Verification items for the finished model (mm, model axes). Face numbers are marked on the shaded views. A direction names the side the tool comes from. Coordinates: 2 decimals unless noted, no trailing zeros. Write each loop counter-clockwise with the first axis right and the second up, starting at its lowest first coordinate (ties: lowest second). Pieces come first, ordered by that corner, then holes. Notation, with made-up numbers: (61.5, 7) -> (105.5, 7) arc R20 ccw to (105.5, 13) -> close; hole circle Ø6 at (80, 49). An arc over 180 degrees is marked (long way). Use a Markdown table: item, result. Add a question column.
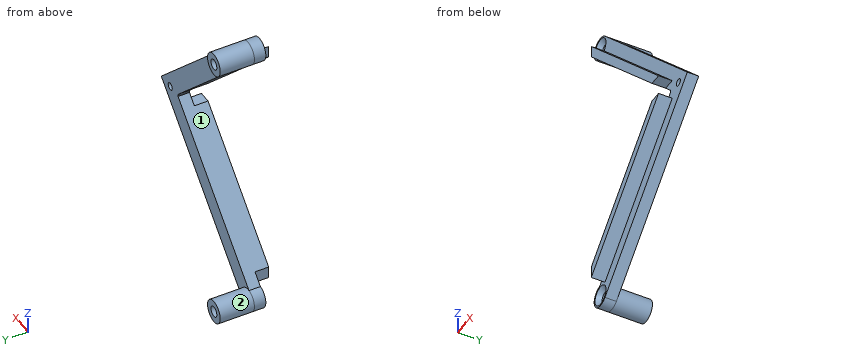
Autodesk Inventor part; units mm, degrees
ref_plane "Work Plane1" through (0, -3.81, 0) normal (0, 1, 0) x (1, 0, 0)
ref_plane "YZ Plane" through (0, 0, 0) normal (1, 0, 0) x (0, 1, 0)
ref_plane "XZ Plane" through (0, 0, 0) normal (0, 1, 0) x (-1, 0, 0)
sketch "Sketch1" plane through (0, 0, 0) normal (0, 1, 0) x (-1, 0, 0)
  line L0 (-41.3092, 0) -> (0, 41.3092)
  circle A0 centre (-36.8191, 0) radius 1.016
  arc A1 (-32.8821, 0) -> (-34.0352, 2.7839) centre (-36.8191, 0) ccw
  line L1 (0, 41.3092) -> (2.2451, 39.0641)
  arc A2 (0, 36.8191) -> (0, 41.3092) centre (2.2451, 39.0641) ccw
  circle A3 centre (2.2451, 39.0641) radius 1.4732
  line L2 (0, 36.8191) -> (-34.0352, 2.7839)
  line L3 (0, 0) -> (-14.0183, 0)
  line L4 (-41.3092, 0) -> (0, -41.3092)
  circle A4 centre (-36.8191, 0) radius 1.016
  arc A5 (-34.0352, -2.7839) -> (-32.8821, 0) centre (-36.8191, 0) ccw
  line L5 (0, -41.3092) -> (2.2451, -39.0641)
  arc A6 (0, -41.3092) -> (0, -36.8191) centre (2.2451, -39.0641) ccw
  circle A7 centre (2.2451, -39.0641) radius 1.4732
  line L6 (0, -36.8191) -> (-34.0352, -2.7839)
  dimension "d0" = 3.175
  dimension "d1" = 58.42
  dimension "d2" = 45
  dimension "d3" = 2.9464
  dimension "d4" = 3.175
  dimension "d5" = 3.937
  dimension "d6" = 2.032
  dimension "d7" = 45
extrude "Extrusion1" add sketch "Sketch1" along normal blind 3.175
sketch "Sketch2" plane through (0, 3.175, 0) normal (0, 1, 0) x (1, 0, 0)
  circle A0 centre (-2.2451, -39.0641) radius 1.4732
  circle A1 centre (-2.2451, -39.0641) radius 3.175
  circle A2 centre (-2.2451, 39.0641) radius 1.4732
  circle A3 centre (-2.2451, 39.0641) radius 3.175
  point P0 (0, 0)
  dimension "d10" = 6.35
  dimension "d11" = 6.35
extrude "Extrusion2" add sketch "Sketch2" along normal blind 9.525
chamfer "Chamfer1" distance 1.27 angle 45 2 edges at (-0.7719, 0, 39.0641) (-0.7719, 0, -39.0641)
sketch "Sketch3" plane through (0, 3.175, 0) normal (0, 1, 0) x (1, 0, 0)
  arc A0 (0, -36.8191) -> (0, -41.3092) centre (-2.2451, -39.0641) ccw
  line L0 (34.0352, -2.7839) -> (0, -36.8191)
  arc A1 (34.0352, 2.7839) -> (34.0352, -2.7839) centre (36.8191, 0) ccw
  line L1 (0, 36.8191) -> (34.0352, 2.7839)
  arc A2 (0, 41.3092) -> (0, 36.8191) centre (-2.2451, 39.0641) ccw
  line L2 (-2.6941, -35.921) -> (32.896, -0.331)
  arc A3 (34.0352, 2.7839) -> (34.0352, -2.7839) centre (36.8191, 0) ccw
  line L3 (32.896, 0.331) -> (-2.6941, 35.921)
  point P0 (0, 0)
  dimension "d17" = 2.54
  dimension "d18" = 2.54
ref_plane "Work Plane1" through (0, -3.81, 0) normal (0, 1, 0) x (1, 0, 0)
extrude "Extrusion3" add sketch "Sketch3" against normal up to surface (3.175 mm away)
sketch "Sketch4" plane through (0, 0, 0) normal (0, -1, 0) x (1, 0, 0)
  line L0 (0, -36.8191) -> (34.0352, -2.7839)
  line L1 (0, 36.8191) -> (34.0352, 2.7839)
  line L2 (-2.6941, -35.921) -> (32.896, -0.331)
  line L3 (-1.6524, -34.8793) -> (32.0954, -1.1315)
  line L4 (32.0954, -1.1315) -> (33.7478, -2.7839)
  line L5 (33.7478, -2.7839) -> (0, -36.5317)
  line L6 (0, -36.5317) -> (-1.6524, -34.8793)
  line L7 (0, 0) -> (11.5163, 0)
  line L8 (-1.6524, 34.8793) -> (32.0954, 1.1315)
  line L9 (32.0954, 1.1315) -> (33.7478, 2.7839)
  line L10 (33.7478, 2.7839) -> (0, 36.5317)
  line L11 (0, 36.5317) -> (-1.6524, 34.8793)
  dimension "d22" = 0.2032
  dimension "d23" = 0.2032
  dimension "d24" = 0.2032
extrude "Extrusion4" add sketch "Sketch4" along normal up to surface (3.81 mm away)
chamfer "Chamfer2" distance 2.3368 angle 45 4 edges at (-1.6524, -1.905, -34.8793) (-1.6524, -1.905, 34.8793) (32.0954, -1.905, 1.1315) (32.0954, -1.905, -1.1315)
properties part number "WIDE SCREEN HOLDER 2SCREEN"
1) Cross-section at B-B on y = 9. Record the boundary of the cut face in (x, z) (3 decimals), then the cut area to 3 significant figures.
2) Thickness scan on L1, parallel to Z at x = -2.5, y = 2.75; L2, parallel to Z at x = 12, y = 1.5; L3, parallel to Z at x = 4.5, y = 2.5. Record the ranges inside material, lowest first.
3) Cross-section at A-A on x = 6. Record the boundary of the cut face in (y, z) (3 decimals).
4) Gauge pin test, flat ends, axial feed: pin 1 (1 mm diameter, centred on x = 1, y = -1.5, fed in from +Z); pin 2 (2.5 mm diameter, centred on x = 36.82, z = 0, fed in from +Y) (3 decimals); pin 3 (1 mm diameter, centred on y = -1.5, z = 34.5, fed in from -X); pin 4 (2.5 mm diameter, centred on x = -2.25, z = 39.06, fed in from -Y). Record the tip position at first contact, or that the pin passes through.
5) Cross-section at C-C on z = 15. Record the boundary of the cut face in (x, y) (3 decimals).
6) Set-up check for the marked faces 1 and 2: record each of +Z, -Z, +X, -X, +Y, -Y from which the full face is reachable in a straight line by a thin tool's end or side.
Returned:
| question | item | result |
|---|---|---|
| 1 | outline | circle Ø6.35 at (-2.245, -39.064); circle Ø6.35 at (-2.245, 39.064); hole circle Ø2.946 at (-2.245, -39.064); hole circle Ø2.946 at (-2.245, 39.064) |
| 1 | area | 49.7 mm² |
| 2 | L1 | z = -42.23 to -40.52, -37.61 to -35.73, 35.73 to 37.61, 40.52 to 42.23 |
| 2 | L2 | z = -29.31 to -21.23, 21.23 to 29.31 |
| 2 | L3 | z = -36.81 to -28.73, 28.73 to 36.81 |
| 3 | outline | (-3.81, -30.532) -> (0, -30.532) -> (0, -35.309) -> (3.175, -35.309) -> (3.175, -27.227) -> (-3.81, -27.227) -> close; (-3.81, 27.227) -> (3.175, 27.227) -> (3.175, 35.309) -> (0, 35.309) -> (0, 30.532) -> (-3.81, 30.532) -> close |
| 4 | pin 1 | stops at z = 36.03 |
| 4 | pin 2 | stops at y = 3.175 |
| 4 | pin 3 | stops at x = 0 |
| 4 | pin 4 | passes through |
| 5 | outline | (18.227, -3.81) -> (21.532, -3.81) -> (21.532, 0) -> (26.309, 0) -> (26.309, 3.175) -> (18.227, 3.175) -> close |
| 6 | face 1 | -X, +Y, -Y |
| 6 | face 2 | +Y |
